Verification items for this drawing (mm, ordinates from the low corner). Round coordinates to 2 decimals unless told otherwise and drop trailing zeros. Loops run counter-clockwise (first coordinate to the right, second up) from the corner with the lowest first, then second, coordinate; pieces in that order, holes last. Notation, with made-up numbers: (-21, 21) - (-5, 21) arc R23 cw to (-5, 47) - close; hole circle Ø3 at (44.5, 77). An arc over 180 degrees is marked (long way). Put each result on its own line as item: value.
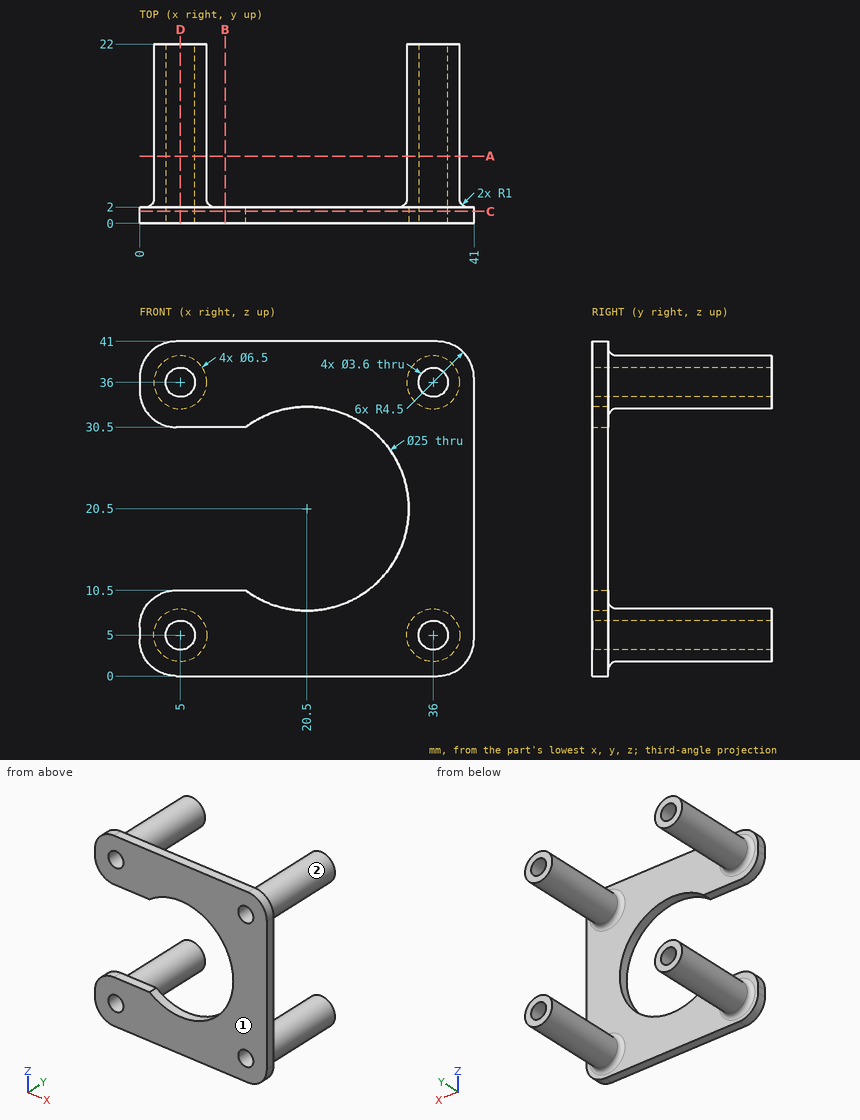
Item 1: Release check for a two-part mould opening along Z. For the marked faces 1 and 2 record: +Z half, -Z half, draft (parallel to the pull), parting line (faces both ways), or undercut.
Filled sheet:
face 1: draft
face 2: undercut
Item 2: Section check C-C on y = 1.5. Enter the section's corners in (x, z).
Filled sheet:
outline: (0, 4.5) arc R4.5 ccw to (4.5, 0) - (36.5, 0) arc R4.5 ccw to (41, 4.5) - (41, 36.5) arc R4.5 ccw to (36.5, 41) - (4.5, 41) arc R4.5 ccw to (0, 36.5) - (0, 35) arc R4.5 ccw to (4.5, 30.5) - (13, 30.5) arc R12.5 cw (long way) to (13, 10.5) - (4.5, 10.5) arc R4.5 ccw to (0, 6) - close; hole circle Ø3.6 at (5, 5); hole circle Ø3.6 at (5, 36); hole circle Ø3.6 at (36, 5); hole circle Ø3.6 at (36, 36)
Item 3: Go/stop test with flat-tipped pins: pin 1 (2 mm diameter, centred on x = 5, z = 5, fed in from -Y); pin 2 (12 mm diameter, centred on y = 13, z = 5.5, fed in from +X); pin 3 (6 mm diameter, centred on x = 31, y = 18, fed in from +Z); pin 4 (10 mm diameter, centred on y = 11.5, z = 31, fed in from -X). Record where each tip stops, or that it passes through.
Filled sheet:
pin 1: through
pin 2: x = 39.25
pin 3: z = 38.56
pin 4: x = 1.75
Item 4: Thickness scan on line 1 (Z direction, x = 36, y = 8); line 2 (Y direction, x = 36, z = 15.5). Record the ranges inside material, lowest first. Write a range as from..to.
Filled sheet:
line 1: 1.75..3.2, 6.8..8.25, 32.75..34.2, 37.8..39.25
line 2: 0..2
Item 5: Section check A-A on y = 8.25. Enter the section's corners in (x, z).
Filled sheet:
outline: circle Ø6.5 at (5, 5); circle Ø6.5 at (5, 36); circle Ø6.5 at (36, 5); circle Ø6.5 at (36, 36); hole circle Ø3.6 at (5, 5); hole circle Ø3.6 at (5, 36); hole circle Ø3.6 at (36, 5); hole circle Ø3.6 at (36, 36)
Item 6: Section check B-B on x = 10.5. Enter the section's corners in (y, z), then the cut area to 3 significant figures.
Filled sheet:
outline: (0, 0) - (2, 0) - (2, 10.5) - (0, 10.5) - close; (0, 30.5) - (2, 30.5) - (2, 41) - (0, 41) - close
area: 42.0 mm²
Item 7: Section check D-D on x = 5. Enter the section's corners in (y, z).
Filled sheet:
outline: (0, 0) - (2, 0) - (2, 0.75) arc R1 cw to (3, 1.75) - (22, 1.75) - (22, 3.2) - (0, 3.2) - close; (0, 6.8) - (22, 6.8) - (22, 8.25) - (3, 8.25) arc R1 cw to (2, 9.25) - (2, 10.5) - (0, 10.5) - close; (0, 30.5) - (2, 30.5) - (2, 31.75) arc R1 cw to (3, 32.75) - (22, 32.75) - (22, 34.2) - (0, 34.2) - close; (0, 37.8) - (22, 37.8) - (22, 39.25) - (3, 39.25) arc R1 cw to (2, 40.25) - (2, 41) - (0, 41) - close
